Can you work these out from the model? Positions are in its coordinate system, mm. Face numbers are marked on the shaded views. A direction names the side the tool comes from. Give positions to 0.01 mm unless a question says otherwise; leave off trailing zeros. Loops run counter-clockwise (first coordinate to the right, second up) from the corner with the lowest first, then second, coordinate; pieces in that order, holes last. Notation, with made-up numbers: M -32.75,23.5 L -13.75,23.5 A12 cw -13.75,32.5 Z; hole C -39,70.25 d5. An arc over 180 degrees is marked long. Use CSV: the item, a comma, the result in double quotes.
from build123d import *

# Parameters (mm, degrees)
F0_W     = 46.6
F0_H     = 27.6
F0_W_2   = 45
F0_H_2   = 26
F1_DEPTH = 77
F2_W     = 46.6
F2_H     = 27.6
F3_DEPTH = 5
F4_W     = 34
F4_H     = 72
F5_DEPTH = 0.8
F6_R     = 3


with BuildPart() as f1:
    # F0 (on Top) → F1 (new body)
    with BuildSketch(Plane.XY):
        Rectangle(F0_W, F0_H)
        Rectangle(F0_W_2, F0_H_2, mode=Mode.SUBTRACT)
    extrude(amount=F1_DEPTH)

    # F2 (on face) → F3 (join)
    with BuildSketch(Plane(origin=(0, 0, 0), x_dir=(1, 0, 0), z_dir=(0, 0, -1))):
        Rectangle(F2_W, F2_H)
    extrude(amount=-F3_DEPTH)

    # F4 (on face) → F5 (cut, through all)
    with BuildSketch(Plane.XZ.offset(13.8)):
        with Locations((0, 41)):
            Rectangle(F4_W, F4_H)
    extrude(amount=-F5_DEPTH, mode=Mode.SUBTRACT)

    # F6
    f6_edges = [f1.edges().sort_by_distance(p)[0] for p in [
        (-17, -13.4, 77),
        (17, -13.4, 77),
        (-17, -13.4, 5),
        (17, -13.4, 5),
    ]]
    fillet(f6_edges, radius=F6_R)


solid = f1.part
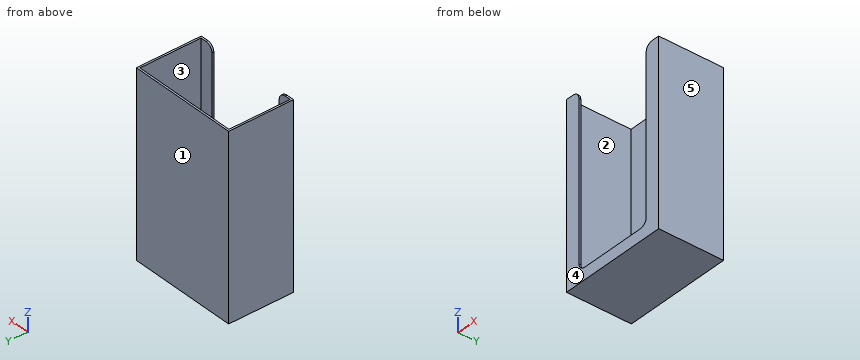
Q1. I want a section at B-B, the plane z = 55.5. Please give me the cut outline in (x, y).
Model answer:
outline,"M -23.3,-13.8 L -17,-13.8 L -17,-13 L -22.5,-13 L -22.5,13 L 22.5,13 L 22.5,-13 L 17,-13 L 17,-13.8 L 23.3,-13.8 L 23.3,13.8 L -23.3,13.8 Z"
Q2. Please list where these lines run through material, in increasing order: L1, parallel to X at y = 6.75, z = 34.5; L2, parallel to Y at x = 19.5, z = 31.5; L3, parallel to Z at x = -14.5, y = 3.25. Write a range as from..to.
Model answer:
L1,"-23.3..-22.5, 22.5..23.3"
L2,"-13.8..-13, 13..13.8"
L3,"0..5"
Q3. If we mould it in two halves opening along Y, with no side actions, what happens to the marked faces 3, 4 and 5? For each: released by +Y, released by -Y, zero draft, split by the parting line, or undercut.
Model answer:
face 3,"undercut"
face 4,"released by -Y"
face 5,"zero draft"
Q4. I want a section at C-C, the plane x = 0.5. Please give me the cut outline in (y, z).
Model answer:
outline,"M -13.8,0 L 13.8,0 L 13.8,77 L 13,77 L 13,5 L -13.8,5 Z"
Q5. For the marked faces 1 and 2, which set-ups out of +Z, -Z, +X, -X, +Y, -Y let a thin tool reach every point of the face, with its end or its side?
Model answer:
face 1,"+Z, -Z, +X, -X, +Y"
face 2,"+Z"
Q6. I want a section at A-A, the plane y = -0.25. Please give me the cut outline in (x, z), then the cut area to 3 significant figures.
Model answer:
outline,"M -23.3,0 L 23.3,0 L 23.3,77 L 22.5,77 L 22.5,5 L -22.5,5 L -22.5,77 L -23.3,77 Z"
area,"348 mm2"
Q7. I'm going to push flat-ended pins straight in: P1, Ø3, axis at x = -11, y = -1, coming from the +Z side; P2, Ø13.5, axis at x = 8, z = 23, coming from the -Y side. Where does each tip first touch, or does it pass through?
Model answer:
P1,"z = 5"
P2,"y = 13"
